Input: dimensioned drawing with shaded views. Units: mm. Origin: part minimum x, y, z. A direction names the side the tool comes from. Give positions to 0.01 mm unless a question says otherwise; leave off trailing zeros. Write each loop counter-clockwise with the first axis right and the second up, starting at its lowest first coordinate (ties: lowest second). Pieces come first, ordered by that corner, then holes. Notation, with made-up numbers: (-7.75, 8) - (35.25, 8) arc R33 cw to (35.25, 38) - close; hole circle Ø9 at (-7.5, 1). An arc over 180 degrees is marked (long way). Answer as a JSON object with one key per item and string values. Group by question number.
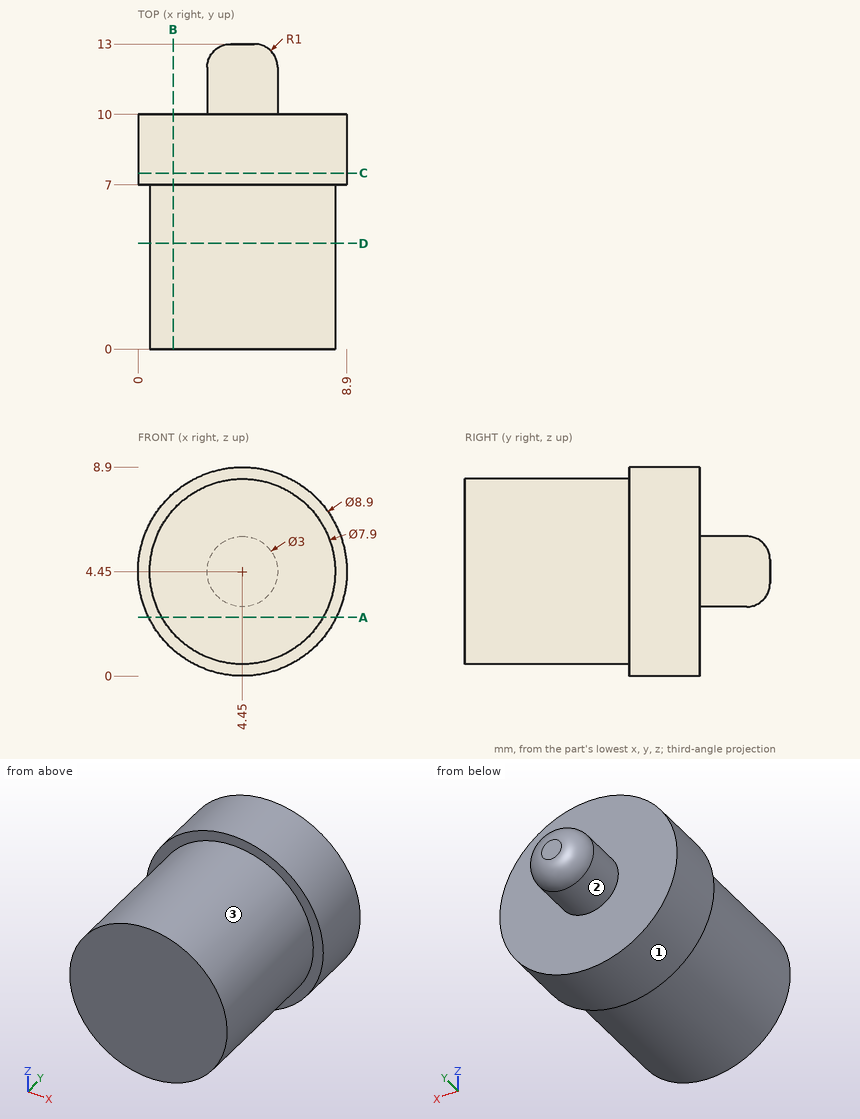
1) Cut plane A-A on z = 2.5. Return the cut outline in (x, y).
2) Cut plane B-B on x = 1.5. Return the cut outline in (y, z), and give its area (3 significant figures).
3) Pin query (flat end, axial travel): P1, Ø3, axis at x = 7, y = 9, coming from the -Z side; P2, Ø1.5, axis at y = 2.5, z = 4, coming from the -X side. Return the tip coordinate at first contact, or that it passes through.
4) Line query: line 1 along Y through (x, z) = (6, 5.5); line 2 along Y through (x, z) = (3.5, 0.5); line 3 along Z through (x, y) = (6, 1.75). Output: solid intervals per line, ascending. Write a range as from..to.
5) Reachability of the marked faces 1, 2 and 3 from +Z, -Z, +X, -X, +Y, -Y: full face, straight path, thin tool, end or side. Return the list, or none.
6) Cut plane D-D on y = 4.5. Return the cut outline in (x, z).
7) Cut plane C-C on y = 7.5. Return the cut outline in (x, z), and give its area (3 significant figures).
Filled in:
{
 "1": {"outline": "(0.45, 7) - (1.01, 7) - (1.01, 0) - (7.89, 0) - (7.89, 7) - (8.45, 7) - (8.45, 10) - (0.45, 10) - close"},
 "2": {"outline": "(0, 1.82) - (7, 1.82) - (7, 1.12) - (10, 1.12) - (10, 7.78) - (7, 7.78) - (7, 7.08) - (0, 7.08) - close", "area": "56.8 mm²"},
 "3": {"P1": "stops at z = 0.13", "P2": "stops at x = 0.5"},
 "4": {"line 1": "y = 0..10", "line 2": "y = 7..10", "line 3": "z = 0.82..8.08"},
 "5": {"face 1": "+Y, -Y", "face 2": "+Y", "face 3": "-Y"},
 "6": {"outline": "circle Ø7.9 at (4.45, 4.45)"},
 "7": {"outline": "circle Ø8.9 at (4.45, 4.45)", "area": "62.2 mm²"}
}
